```python
from build123d import *

# Parameters (mm, degrees)
F0_W     = 134.842023
F0_H     = 109.384302
F0_W_2   = 17.344825
F0_H_2   = 17.065071
F1_DEPTH = 63.5
F2_R     = 12.7
F3_R     = 20.174327
F4_DEPTH = 87.63


with BuildPart() as f1:
    # F0 (on Front) → F1 (new body)
    with BuildSketch(Plane.XZ):
        with Locations((-0.380561, 8.672414)):
            Rectangle(F0_W, F0_H)
        with Locations((-37.588007, 29.374301)):
            Rectangle(F0_W_2, F0_H_2, mode=Mode.SUBTRACT)
    extrude(amount=F1_DEPTH)

    # F2
    f2_edges = [f1.edges().sort_by_distance(p)[0] for p in [
        (67.040451, -31.75, 63.364565),
    ]]
    fillet(f2_edges, radius=F2_R)

    # F3 (on face) → F4 (join)
    with BuildSketch(Plane.XY.offset(63.364565)):
        with Locations((-20.378303, -31.75)):
            Circle(F3_R)
    extrude(amount=F4_DEPTH)


solid = f1.part
```
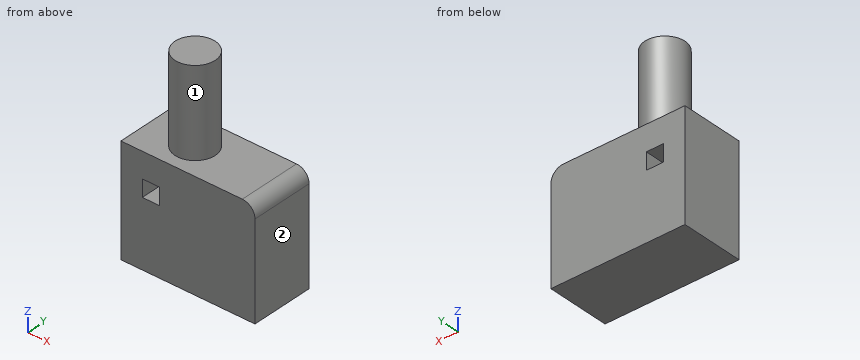
Model file for the job. Use its own axes, mm. Face numbers are marked on the shaded views. A direction names the side the tool comes from. Coordinates: 2 decimals unless noted, no trailing zeros. Loops run counter-clockwise (first coordinate to the right, second up) from the corner with the lowest first, then second, coordinate; pieces in that order, holes last. Notation, with made-up numbers: (86.5, 31.5) -> (131.5, 31.5) arc R33 ccw to (131.5, 69.5) -> close; hole circle Ø1 at (-23.5, 28). An arc over 180 degrees is marked (long way). Answer as a JSON object with one key per item and string values.
Q1. 3-axis set-ups, long thin cutter, end or side, ignore diameter. For the marked faces 1 and 2: which of +Z, -Z, +X, -X, +Y, -Y reach the whole face in a straight line?
Report:
{"face 1": "+Z", "face 2": "+Z, -Z, +X, +Y, -Y"}
Q2. Cut at B-B (y = -31.75). List the corners of the cut face in (x, z), and give its area (3 significant figures).
Report:
{"outline": "(-67.8, -46.02) -> (67.04, -46.02) -> (67.04, 50.66) arc R12.7 ccw to (54.34, 63.36) -> (-0.2, 63.36) -> (-0.2, 150.99) -> (-40.55, 150.99) -> (-40.55, 63.36) -> (-67.8, 63.36) -> close; hole (-46.26, 20.84) -> (-28.92, 20.84) -> (-28.92, 37.91) -> (-46.26, 37.91) -> close", "area": "18,000 mm2"}
Q3. Flat gauge pins, fed straight in: P1, Ø12, axis at x = 3, y = -39.5, coming from the +Z side; P2, Ø4, axis at y = -11.5, z = 90, coming from the +X side. Where does each tip first touch, or does it go through?
Report:
{"P1": "stops at z = 150.99", "P2": "stops at x = -11.78"}
Q4. Cut at C-C (x = -50.5). List the corners of the cut face in (y, z).
Report:
{"outline": "(-63.5, -46.02) -> (0, -46.02) -> (0, 63.36) -> (-63.5, 63.36) -> close"}
Q5. Cut at D-D (y = -45). List the corners of the cut face in (x, z).
Report:
{"outline": "(-67.8, -46.02) -> (67.04, -46.02) -> (67.04, 50.66) arc R12.7 ccw to (54.34, 63.36) -> (-5.17, 63.36) -> (-5.17, 150.99) -> (-35.59, 150.99) -> (-35.59, 63.36) -> (-67.8, 63.36) -> close; hole (-46.26, 20.84) -> (-28.92, 20.84) -> (-28.92, 37.91) -> (-46.26, 37.91) -> close"}
Q6. Probe probe 1 along X at (y, z) = (-11, 23.5); probe 2 along Z at (x, y) = (52.5, -59); probe 3 along Z at (x, y) = (55, -50). List the from-to ranges inside material, lowest first.
Report:
{"probe 1": "x = -67.8 to -46.26, -28.92 to 67.04", "probe 2": "z = -46.02 to 63.36", "probe 3": "z = -46.02 to 63.35"}
Q7. Cut at A-A (y = -9). List the corners of the cut face in (x, z), and give its area (3 significant figures).
Report:
{"outline": "(-67.8, -46.02) -> (67.04, -46.02) -> (67.04, 50.66) arc R12.7 ccw to (54.34, 63.36) -> (-67.8, 63.36) -> close; hole (-46.26, 20.84) -> (-28.92, 20.84) -> (-28.92, 37.91) -> (-46.26, 37.91) -> close", "area": "14,400 mm2"}
